from build123d import *

# Parameters (mm, degrees)
SKETCH_5_R      = 5
EXTRUDE_1_DEPTH = 0.8


with BuildPart() as part:
    # Sketch 5 → Extrude 1 (new body)
    with BuildSketch(Plane(origin=(0, 0, 0), x_dir=(1, 0, 0), z_dir=(0, 1, 0))):
        Polygon((-13, -23.5), (-13, -14.6), (-12, -14.6), (-12, -13), (-8, -13), (-8, -14.6), (8, -14.6), (8, -13), (12, -13), (12, -14.6), (13, -14.6), (13, -23.5), (15, -23.5), (15, -21.5), (17, -21.5), (17, -19.5), (27, -19.5), (27, -17.5), (29, -17.5), (29, -15.5), (31, -15.5), (31, -13.5), (33, -13.5), (33, -9.5), (31, -9.5), (31, 9.5), (33, 9.5), (33, 13.5), (31, 13.5), (31, 15.5), (29, 15.5), (29, 17.5), (27, 17.5), (27, 19.5), (17, 19.5), (17, 21.5), (15, 21.5), (15, 23.5), (13, 23.5), (13, 14.6), (12, 14.6), (12, 13), (8, 13), (8, 14.6), (-8, 14.6), (-8, 13), (-12, 13), (-12, 14.6), (-13, 14.6), (-13, 23.5), (-26, 23.5), (-26, 21.5), (-28, 21.5), (-28, 19.5), (-30, 19.5), (-30, 17.5), (-32, 17.5), (-32, 15.5), (-34, 15.5), (-34, 13.5), (-36, 13.5), (-36, 11.5), (-38, 11.5), (-38, 9.5), (-40, 9.5), (-40, -9.5), (-38, -9.5), (-38, -11.5), (-36, -11.5), (-36, -13.5), (-34, -13.5), (-34, -15.5), (-32, -15.5), (-32, -17.5), (-30, -17.5), (-30, -19.5), (-28, -19.5), (-28, -21.5), (-26, -21.5), (-26, -23.5), align=None)
        with Locations(Location((-14, 0, 0), (0, 0, 270))):
            Circle(SKETCH_5_R, mode=Mode.SUBTRACT)
        Polygon((-17.728524487, -17.009831185), (-17.241222705, -20.415141299), (-15.756349109, -20.202655057), (-16.243650891, -16.797344943), align=None, mode=Mode.SUBTRACT)
        Polygon((-23.763263852, -12.051103665), (-23.19560882, -15.443944328), (-21.716172484, -15.196420332), (-22.283827516, -11.803579668), align=None, mode=Mode.SUBTRACT)
        Polygon((-28.776184385, -4.834516937), (-26.354359033, -7.277540056), (-25.289087324, -6.22151156), (-27.710912676, -3.77848844), align=None, mode=Mode.SUBTRACT)
        Polygon((-32.230719309, -4.802671603), (-34.781815362, -2.494965181), (-33.775548026, -1.382568646), (-31.224451974, -3.690275068), align=None, mode=Mode.SUBTRACT)
        Polygon((-17.241222705, 20.415141299), (-15.756349109, 20.202655057), (-16.243650891, 16.797344943), (-17.728524487, 17.009831185), align=None, mode=Mode.SUBTRACT)
        Polygon((-23.19560882, 15.443944328), (-21.716172484, 15.196420332), (-22.283827516, 11.803579668), (-23.763263852, 12.051103665), align=None, mode=Mode.SUBTRACT)
        Polygon((-26.354359033, 7.277540056), (-25.289087324, 6.22151156), (-27.710912676, 3.77848844), (-28.776184385, 4.834516937), align=None, mode=Mode.SUBTRACT)
        Polygon((-34.781815362, 2.494965181), (-33.775548026, 1.382568646), (-31.224451974, 3.690275068), (-32.230719309, 4.802671603), align=None, mode=Mode.SUBTRACT)
    extrude(amount=EXTRUDE_1_DEPTH)


solid = part.part
The listing builds one solid part. Answer for the finished solid, in the listing's coordinates (mm). A direction names the side the tool comes from. Give positions to 0.01 mm unless a question says otherwise; leave off trailing zeros. Order: outer loops, then holes, each group sorted by start corner. A loop starts at its lowest first (then second) coordinate and runs counter-clockwise, first axis right, second up. Notation, with made-up numbers: (-18, 68.25) - (-4, 68.25) arc R18 cw to (-4, 101.25) - close; hole circle Ø10 at (85, 15). An arc over 180 degrees is marked (long way). One line per item, written item: value. Start each with the question number.
1) A cutting plane is placed at C-C on y = 0.3. State how many separate pieces and enclosed holes the cut face has, then the cut area to 3 significant figures.
2) A tool of negligible diameter and unlimited length cuts with its end or side. For faces 3 (the face through (-33.488, 0.394, 3.665)), 4 (the face through (-4, 0, 0)), from which of +Z, -Z, +X, -X, +Y, -Y can it reach the whole face along a straight path? Write none if from no direction.
3) A cutting plane is placed at A-A on x = -14. Give the vertices of the cut face in (y, z), then the cut area to 3 significant figures.
4) The mould has two halves that part along Z. Classify faces 1 (the face through (-27.58, 0.39, 6.04)), 2 (the face through (-4, 0.8, 0)): released by +Z, released by -Z, zero draft, split by the parting line, or undercut.
5) A cutting plane is placed at B-B on z = 0. Give the vertices of the cut face in (x, y), then the cut area to 3 significant figures.
6) Find the intervals of material crossed by L1, parallel to X at y = 0.6, z = 0; L2, parallel to X at y = 0.45, z = -16; L3, parallel to X at y = 0.45, z = -19, in increasing order.
7) A cutting plane is placed at D-D on x = -1. Give the vertices of the cut face in (y, z).
Answer sheet:
1. separate pieces: 1
1. enclosed holes: 9
1. area: 2,380 mm2
2. face 3: +Y, -Y
2. face 4: +Z, -Z, +X, -X, -Y
3. outline: (0, -23.5) - (0.8, -23.5) - (0.8, -5) - (0, -5) - close; (0, 5) - (0.8, 5) - (0.8, 23.5) - (0, 23.5) - close
3. area: 29.6 mm2
4. face 1: undercut
4. face 2: zero draft
5. outline: (-40, 0) - (-19, 0) - (-19, 0.8) - (-40, 0.8) - close; (-9, 0) - (31, 0) - (31, 0.8) - (-9, 0.8) - close
5. area: 48.8 mm2
6. L1: x = -40 to -19, -9 to 31
6. L2: x = -32 to -13, 13 to 29
6. L3: x = -30 to -17.44, -15.93 to -13, 13 to 27
7. outline: (0, -14.6) - (0.8, -14.6) - (0.8, 14.6) - (0, 14.6) - close
